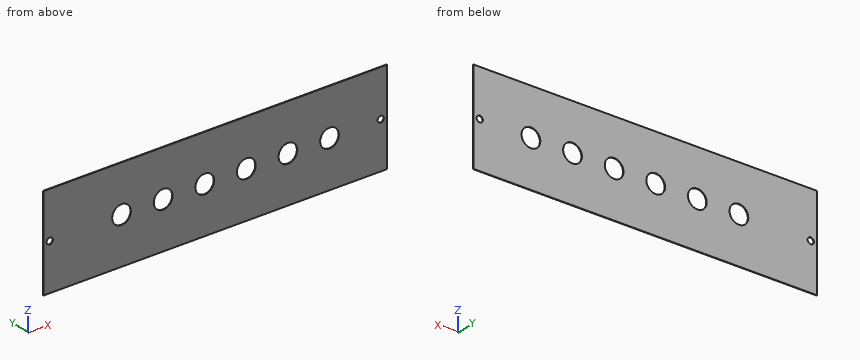
```python
from build123d import *

# Parameters (mm, degrees)
SKETCH1_W          = 550
SKETCH1_H          = 150
BASE_FLANGE1_DEPTH = 1
SKETCH3_R          = 5
CUT_EXTRUDE1_DEPTH = 1
SKETCH4_R          = 15
CUT_EXTRUDE2_DEPTH = 1
LPATTERN1_COUNT    = 6
LPATTERN1_PITCH    = 66.6


# Sheet-metal steps are written as plain solids
with BuildPart() as part:
    # Sketch1 → Base-Flange1 (new body)
    with BuildSketch(Plane(origin=(0, 0, 0), x_dir=(1, 0, 0), z_dir=(0, 1, 0))):
        Rectangle(SKETCH1_W, SKETCH1_H)
    extrude(amount=-BASE_FLANGE1_DEPTH)

    # Sketch3 → Cut-Extrude1 (cut)
    with BuildSketch(Plane(origin=(0, 0, 0), x_dir=(1, 0, 0), z_dir=(0, 1, 0))):
        with Locations(Location((-265, 0, 0), (0, 0, 270))):
            Circle(SKETCH3_R)
        with Locations(Location((265, 0, 0), (0, 0, 270))):
            Circle(SKETCH3_R)
    extrude(amount=-CUT_EXTRUDE1_DEPTH, mode=Mode.SUBTRACT)

    # Sketch4 → Cut-Extrude2 (cut)
    with BuildSketch(Plane.XZ.offset(1)):
        with Locations(Location((-150, 0, 0), (0, 0, 270))):
            Circle(SKETCH4_R)
    cut_extrude2 = extrude(amount=-CUT_EXTRUDE2_DEPTH, mode=Mode.SUBTRACT)

    # LPattern1: Cut-Extrude2 ×6
    with Locations(*[(i * LPATTERN1_PITCH, 0, 0) for i in range(1, LPATTERN1_COUNT)]):
        add(cut_extrude2, mode=Mode.SUBTRACT)


solid = part.part
```
Source: CAD feature listing. Evaluate the final solid. Frame: model axes, mm. Round coordinates to 2 decimals unless told otherwise and drop trailing zeros. Loops run counter-clockwise (first coordinate to the right, second up) from the corner with the lowest first, then second, coordinate; pieces in that order, holes last.
1. Section query B-B on y = -0.35. Give the number of separate pieces and of enclosed holes in the cut face, and give its area (3 significant figures).
2. Ray query, L1, parallel to Z at x = 265, y = -0.75; L2, parallel to Z at x = -29, y = -0.9. Return the intervals inside material, ascending.
3. Contact query for a flat-ended pin moving along its axis: pin 1 (18 mm diameter, centred on x = 49.8, z = 0, fed in from -Y). Output: stop coordinate, or through.
4. Section query C-C on x = -265. Output: boundary loops of the cut face in (y, z), and give its area (3 significant figures).
5. Section query A-A on x = 116.4. Output: boundary loops of the cut face in (y, z).
Answers below:
1. separate pieces: 1
1. enclosed holes: 8
1. area: 78,100 mm2
2. L1: z = -75 to -5, 5 to 75
2. L2: z = -75 to -8.73, 8.73 to 75
3. pin 1: passes through
4. outline: (-1, -75) - (0, -75) - (0, -5) - (-1, -5) - close; (-1, 5) - (0, 5) - (0, 75) - (-1, 75) - close
4. area: 140 mm2
5. outline: (-1, -75) - (0, -75) - (0, -15) - (-1, -15) - close; (-1, 15) - (0, 15) - (0, 75) - (-1, 75) - close
